```python
from build123d import *

# Parameters (mm, degrees)
SKETCH1_W           = 168
SKETCH1_H           = 120
BOSS_EXTRUDE1_DEPTH = 10
CUT_EXTRUDE1_DEPTH  = 104.7111373
CHAMFER1_SIZE       = 8
FILLET1_R           = 2
SKETCH3_W           = 168
SKETCH3_H           = 20
CUT_EXTRUDE2_DEPTH  = 5
SKETCH4_W           = 168
SKETCH4_H           = 20
CUT_EXTRUDE3_DEPTH  = 3
CHAMFER2_SIZE       = 5
SHELL1_START        = -66
SHELL1_DEPTH        = 10.263276069
SHELL1_START_2      = -42
SHELL1_2_DEPTH      = 10.263276069
SHELL1_START_3      = 6
SHELL1_3_DEPTH      = 10.263276069
SHELL1_START_4      = 30
SHELL1_4_DEPTH      = 10.263276069
SHELL1_START_5      = 54
SHELL1_5_DEPTH      = 10.263276069
CUT_EXTRUDE4_DEPTH  = 164.719271926
SKETCH6_R           = 1.75
CUT_EXTRUDE5_DEPTH  = 104.348923555


# Read off the part's stored shape, not the designer's step: Shell1
with BuildPart() as part:
    # Sketch1 → Boss-Extrude1 (new body)
    with BuildSketch(Plane.XY):
        Rectangle(SKETCH1_W, SKETCH1_H)
    extrude(amount=BOSS_EXTRUDE1_DEPTH)

    # Sketch2 → Cut-Extrude1 (cut, through all)
    with BuildSketch(Plane.XY.offset(10)):
        Polygon((-68, 40), (-68, -18), (-53.736723931, -18), (-53.736723931, 40), (-44, 40), (-44, -18), (-29.736723931, -18), (-29.736723931, 40), (4, 40), (4, -18), (18.263276069, -18), (18.263276069, 40), (28, 40), (28, -18), (42.263276069, -18), (42.263276069, 40), (52, 40), (52, -18), (66.263276069, -18), (66.263276069, 40), (84, 40), (84, -60), (-84, -60), (-84, 40), align=None)
    extrude(amount=-CUT_EXTRUDE1_DEPTH, mode=Mode.SUBTRACT)

    # Chamfer1
    chamfer1_edges = [part.edges().sort_by_distance(p)[0] for p in [
        (59.131638035, -18, 10),
        (35.131638035, -18, 10),
        (11.131638035, -18, 10),
        (-36.868361965, -18, 10),
        (-60.868361965, -18, 10),
    ]]
    chamfer(chamfer1_edges, length=CHAMFER1_SIZE)

    # Fillet1
    fillet1_edges = [part.edges().sort_by_distance(p)[0] for p in [
        (66.263276069, 15, 10),
        (42.263276069, 15, 10),
        (18.263276069, 15, 10),
        (-29.736723931, 15, 10),
        (-53.736723931, 15, 10),
        (52, 15, 10),
        (-68, 15, 10),
        (-44, 15, 10),
        (4, 15, 10),
        (28, 15, 10),
    ]]
    fillet(fillet1_edges, radius=FILLET1_R)

    # Sketch3 → Cut-Extrude2 (cut)
    with BuildSketch(Plane.XY.offset(10)):
        with Locations((0, 50)):
            Rectangle(SKETCH3_W, SKETCH3_H)
    extrude(amount=-CUT_EXTRUDE2_DEPTH, mode=Mode.SUBTRACT)

    # Sketch4 → Cut-Extrude3 (cut)
    with BuildSketch(Plane(origin=(0, 0, 0), x_dir=(-1, 0, 0), z_dir=(0, 0, -1))):
        with Locations((0, 50)):
            Rectangle(SKETCH4_W, SKETCH4_H)
    extrude(amount=-CUT_EXTRUDE3_DEPTH, mode=Mode.SUBTRACT)

    # Chamfer2
    # the kernel refuses this chamfer: 5 mm, written as the material it takes off along each edge
    with BuildSketch(Plane(origin=(77.121691009, 40, 10), x_dir=(0, 0.027495876610586317, -0.9996219169112968), z_dir=(-1, 0, 0)), Plane(origin=(53.121691009, 40, 10), x_dir=(0, 0.027495876610586317, -0.9996219169112968), z_dir=(-1, 0, 0)), Plane(origin=(29.121691009, 40, 10), x_dir=(0, 0.027495876610586317, -0.9996219169112968), z_dir=(-1, 0, 0)), Plane(origin=(-18.878308991, 40, 10), x_dir=(0, 0.027495876610586317, -0.9996219169112968), z_dir=(-1, 0, 0))) as chamfer2_piece_1:
        Polygon((CHAMFER2_SIZE * 0.999621916911, CHAMFER2_SIZE * 0.0274958766106), (-CHAMFER2_SIZE * 0.0274958766106, CHAMFER2_SIZE * 0.999621916911), (0, 0), align=None)
    extrude(amount=35.980105949, mode=Mode.SUBTRACT)
    with BuildSketch(Plane(origin=(-42.878308991, 40, 10), x_dir=(0, -0.9996219169112968, 0.027495876610586317), z_dir=(-1, 0, 0))) as chamfer2_piece_2:
        Polygon((CHAMFER2_SIZE * 0.999621916911, -CHAMFER2_SIZE * 0.0274958766106), (-CHAMFER2_SIZE * 0.0274958766106, -CHAMFER2_SIZE * 0.999621916911), (0, 0), align=None)
    extrude(amount=35.980105949, mode=Mode.SUBTRACT)

    # Shell1 outline → Shell1 (cut)
    with BuildSketch(Plane.YZ.offset(SHELL1_START)):
        Polygon((38, 4.171572875), (34.171572875, 8), (-9.171572875, 8), (-16, 1.171572875), (-16, 0), (38, 0), align=None)
    extrude(amount=SHELL1_DEPTH, mode=Mode.SUBTRACT)

    # Shell1 2 outline → Shell1 2 (cut)
    with BuildSketch(Plane.YZ.offset(SHELL1_START_2)):
        Polygon((38, 4.171572875), (34.171572875, 8), (-9.171572875, 8), (-16, 1.171572875), (-16, 0), (38, 0), align=None)
    extrude(amount=SHELL1_2_DEPTH, mode=Mode.SUBTRACT)

    # Shell1 3 outline → Shell1 3 (cut)
    with BuildSketch(Plane.YZ.offset(SHELL1_START_3)):
        Polygon((38, 4.171572875), (34.171572875, 8), (-9.171572875, 8), (-16, 1.171572875), (-16, 0), (38, 0), align=None)
    extrude(amount=SHELL1_3_DEPTH, mode=Mode.SUBTRACT)

    # Shell1 4 outline → Shell1 4 (cut)
    with BuildSketch(Plane.YZ.offset(SHELL1_START_4)):
        Polygon((38, 4.171572875), (34.171572875, 8), (-9.171572875, 8), (-16, 1.171572875), (-16, 0), (38, 0), align=None)
    extrude(amount=SHELL1_4_DEPTH, mode=Mode.SUBTRACT)

    # Shell1 5 outline → Shell1 5 (cut)
    with BuildSketch(Plane.YZ.offset(SHELL1_START_5)):
        Polygon((38, 4.171572875), (34.171572875, 8), (-9.171572875, 8), (-16, 1.171572875), (-16, 0), (38, 0), align=None)
    extrude(amount=SHELL1_5_DEPTH, mode=Mode.SUBTRACT)

    # Sketch5 → Cut-Extrude4 (cut, through all)
    with BuildSketch(Plane.ZY.offset(68)):
        Polygon((3, 40), (0, 31.673069766), (0, 40), align=None)
    extrude(amount=-CUT_EXTRUDE4_DEPTH, mode=Mode.SUBTRACT)

    # Sketch6 → Cut-Extrude5 (cut, through all)
    with BuildSketch(Plane.XY.offset(5)):
        with Locations((-64, 52)):
            Circle(SKETCH6_R)
        with Locations((-34, 52)):
            Circle(SKETCH6_R)
        with Locations((-4, 52)):
            Circle(SKETCH6_R)
        with Locations((26, 52)):
            Circle(SKETCH6_R)
        with Locations((56, 52)):
            Circle(SKETCH6_R)
    extrude(amount=-CUT_EXTRUDE5_DEPTH, mode=Mode.SUBTRACT)


solid = part.part
```
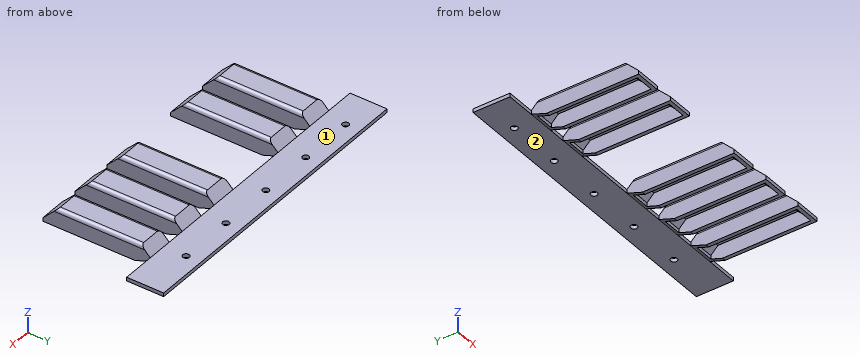
Work out the finished part from the listing and answer in its coordinate system (mm). Face numbers are marked on the shaded views. A direction names the side the tool comes from. Give positions to 0.01 mm unless a question says otherwise; leave off trailing zeros. Order: outer loops, then holes, each group sorted by start corner. A loop starts at its lowest first (then second) coordinate and runs counter-clockwise, first axis right, second up.
1. Section A-A, the plane x = -4 is taken. Determine the outline of the cut face in (y, z), and give its area (3 significant figures).
Result sheet:
outline: (40, 3) - (50.25, 3) - (50.25, 5) - (40, 5) - close; (53.75, 3) - (60, 3) - (60, 5) - (53.75, 5) - close
area: 33.0 mm2
2. Straight lines are drawn through the part: L1, parallel to X at y = 38, z = 4.75; L2, parallel to Y at x = 56, z = 3.65; L3, parallel to Y at x = -41, z = 3.25. For each, find the intervals that lie inside material, in ascending order.
Result sheet:
L1: x = -68 to -53.74, -44 to -29.74, 4 to 18.26, 28 to 42.26, 52 to 66.26
L2: y = -16.35 to -13.52, 38 to 50.25, 53.75 to 60
L3: y = -16.75 to -13.92, 38 to 60
3. Each of these flat-tipped pins is pushed along its axis until it touches: P1, Ø2, axis at y = 23, z = 1.5, coming from the -X side; P2, Ø1.5, axis at x = -38, z = 8, coming from the +Y side; P3, Ø0.6, axis at x = 74.5, z = 4, coming from the -Y side; P4, Ø2, axis at x = -34, y = 52, coming from the -Z side. Where does it stop, or does it pass through?
Result sheet:
P1: stops at x = -68
P2: stops at y = 37.75
P3: stops at y = 40
P4: passes through
4. Section D-D, the plane y = 47.5 is taken. Determine the outline of the cut face in (x, z).
Result sheet:
outline: (-84, 3) - (84, 3) - (84, 5) - (-84, 5) - close
5. For the marked faces 1 and 2, determine the directions among +Z, -Z, +X, -X, +Y, -Y from which every point of the face is accessible in a straight line to the end or side of a thin tool.
Result sheet:
face 1: +Z, +X, -X, +Y
face 2: -Z, +X, -X, +Y
6. Section B-B, the plane y = 2.5 is taken. Give the number of separate pieces and of enclosed holes in the cut face, and give its area (3 significant figures).
Result sheet:
separate pieces: 5
enclosed holes: 0
area: 294 mm2
7. Section C-C, the plane x = -34 is taken. Determine the outline of the cut face in (y, z), and give its area (3 significant figures).
Result sheet:
outline: (-18, 0) - (-16, 0) - (-16, 1.17) - (-9.17, 8) - (34.17, 8) - (38, 4.17) - (38, 2.28) - (40, 3) - (50.25, 3) - (50.25, 5) - (40, 5) - (35, 10) - (-10, 10) - (-18, 2) - close; (53.75, 3) - (60, 3) - (60, 5) - (53.75, 5) - close
area: 162 mm2
